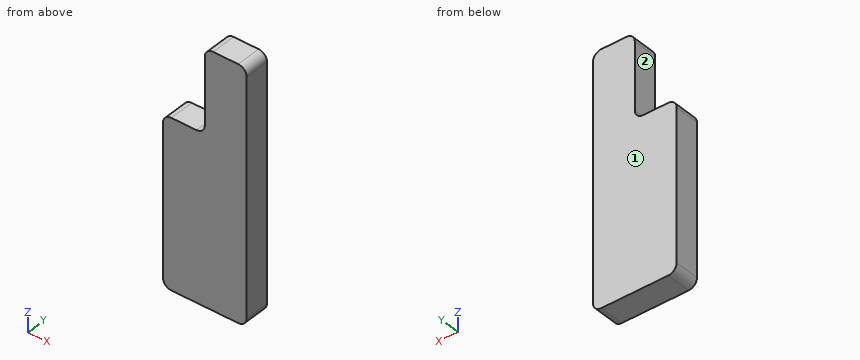
```python
from build123d import *

# Parameters (mm, degrees)
ESBO_O1_W                = 10
ESBO_O1_H                = 30
RESSALTO_EXTRUS_O1_DEPTH = 3
ESBO_O2_W                = 5
ESBO_O2_H                = 10
CORTE_EXTRUS_O1_DEPTH    = 3
FILETE1_R                = 1
FILETE2_R                = 1
FILETE3_R                = 1
FILETE4_R                = 1
FILETE5_R                = 1
FILETE6_R                = 1


with BuildPart() as part:
    # Esboço1 → Ressalto-extrusão1 (new body)
    with BuildSketch(Plane(origin=(0, 0, 0), x_dir=(1, 0, 0), z_dir=(0, 1, 0))):
        Rectangle(ESBO_O1_W, ESBO_O1_H)
    extrude(amount=RESSALTO_EXTRUS_O1_DEPTH)

    # Esboço2 → Corte-extrusão1 (cut)
    with BuildSketch(Plane(origin=(0, 3, 0), x_dir=(1, 0, 0), z_dir=(0, 1, 0))):
        with Locations((-2.5, -10)):
            Rectangle(ESBO_O2_W, ESBO_O2_H)
    extrude(amount=-CORTE_EXTRUS_O1_DEPTH, mode=Mode.SUBTRACT)

    # Filete1
    filete1_edges = [part.edges().sort_by_distance(p)[0] for p in [
        (5, 1.5, 15),
    ]]
    fillet(filete1_edges, radius=FILETE1_R)

    # Filete2
    filete2_edges = [part.edges().sort_by_distance(p)[0] for p in [
        (0, 1.5, 15),
    ]]
    fillet(filete2_edges, radius=FILETE2_R)

    # Filete3
    filete3_edges = [part.edges().sort_by_distance(p)[0] for p in [
        (0, 1.5, 5),
    ]]
    fillet(filete3_edges, radius=FILETE3_R)

    # Filete4
    filete4_edges = [part.edges().sort_by_distance(p)[0] for p in [
        (-5, 1.5, 5),
    ]]
    fillet(filete4_edges, radius=FILETE4_R)

    # Filete5
    filete5_edges = [part.edges().sort_by_distance(p)[0] for p in [
        (-5, 1.5, -15),
    ]]
    fillet(filete5_edges, radius=FILETE5_R)

    # Filete6
    filete6_edges = [part.edges().sort_by_distance(p)[0] for p in [
        (5, 1.5, -15),
    ]]
    fillet(filete6_edges, radius=FILETE6_R)


solid = part.part
```
The listing builds one solid part. Answer for the finished solid, in the listing's coordinates (mm). Face numbers are marked on the shaded views. A direction names the side the tool comes from. Give positions to 0.01 mm unless a question says otherwise; leave off trailing zeros. Loops run counter-clockwise (first coordinate to the right, second up) from the corner with the lowest first, then second, coordinate; pieces in that order, holes last. Notation, with made-up numbers: (17, 13.25) - (76, 13.25) arc R3 ccw to (76, 18.25) - close; hole circle Ø10 at (67, -18). An arc over 180 degrees is marked (long way). Return JSON: item names as keys, results as strings. Group by question number.
1. Find section B-B (z = 12.25). Write down the section's boundary in (x, y), then the cut area to 3 significant figures.
2. Straight lines are drawn through the part: line 1 (X direction, y = 1.1, z = 11.5); line 2 (Z direction, x = -2.75, y = 1.45); line 3 (Z direction, x = -0.5, y = 1.7). For each, find the intervals that lie inside material, in ascending order. Write a range as [from, to].
3. Which of the six approach directions +Z, -Z, +X, -X, +Y, -Y give full straight-line access (tool end or side, diameter ignored) to the marked faces 1 and 2?
4. Find section C-C (x = -3.25). Write down the section's boundary in (y, z).
5. Find section A-A (y = 1.5). Write down the section's boundary in (x, z).
Verdict:
{
 "1": {"outline": "(0, 0) - (5, 0) - (5, 3) - (0, 3) - close", "area": "15.0 mm^2"},
 "2": {"line 1": "x = [0, 5]", "line 2": "z = [-15, 5]", "line 3": "z = [-15, 5.13]"},
 "3": {"face 1": "+Z, -Z, +X, -X, +Y", "face 2": "+Z, -X, +Y, -Y"},
 "4": {"outline": "(0, -15) - (3, -15) - (3, 5) - (0, 5) - close"},
 "5": {"outline": "(-5, -14) arc R1 ccw to (-4, -15) - (4, -15) arc R1 ccw to (5, -14) - (5, 14) arc R1 ccw to (4, 15) - (1, 15) arc R1 ccw to (0, 14) - (0, 6) arc R1 cw to (-1, 5) - (-4, 5) arc R1 ccw to (-5, 4) - close"}
}
